from build123d import *

# Parameters (mm, degrees)
SKETCH1_R           = 15
SKETCH1_R_2         = 10.05
BOSS_EXTRUDE1_DEPTH = 6
SKETCH3_R           = 2.95
CUT_EXTRUDE1_DEPTH  = 3
CIRPATTERN1_COUNT   = 3
SKETCH4_R           = 1.65
CUT_EXTRUDE2_DEPTH  = 11
CIRPATTERN3_COUNT   = 3


with BuildPart() as part:
    # Sketch1 → Boss-Extrude1 (new body)
    with BuildSketch(Plane(origin=(0, 0, 0), x_dir=(0, 0, -1), z_dir=(1, 0, 0))):
        Circle(SKETCH1_R)
        Circle(SKETCH1_R_2, mode=Mode.SUBTRACT)
    extrude(amount=BOSS_EXTRUDE1_DEPTH)

    # Sketch3 → Cut-Extrude1 (cut)
    with BuildSketch(Plane(origin=(0, -7.5, 12.990381057), x_dir=(1, 0, 0), z_dir=(0, -0.5000000000000044, 0.866025403784436))):
        with Locations(Location((3, 0, 0), (0, 0, 270))):
            Circle(SKETCH3_R)
    cut_extrude1 = extrude(amount=-CUT_EXTRUDE1_DEPTH, mode=Mode.SUBTRACT)

    # CirPattern1: Cut-Extrude1 ×3 about axis
    cirpattern1_axis = Axis((0, 0, 0), (1, 0, 0))
    for i in range(1, CIRPATTERN1_COUNT):
        add(cut_extrude1.rotate(cirpattern1_axis, i * 360 / CIRPATTERN1_COUNT), mode=Mode.SUBTRACT)

    # Sketch4 → Cut-Extrude2 (cut)
    with BuildSketch(Plane(origin=(0, -7.5, 12.990381057), x_dir=(1, 0, 0), z_dir=(0, -0.5000000000000044, 0.866025403784436))):
        with Locations(Location((3, 0, 0), (0, 0, 270))):
            Circle(SKETCH4_R)
    cut_extrude2 = extrude(amount=-CUT_EXTRUDE2_DEPTH, mode=Mode.SUBTRACT)

    # CirPattern3: Cut-Extrude2 ×3 about axis
    cirpattern3_axis = Axis((6, 0, 0), (-1, 0, 0))
    for i in range(1, CIRPATTERN3_COUNT):
        add(cut_extrude2.rotate(cirpattern3_axis, i * 360 / CIRPATTERN3_COUNT), mode=Mode.SUBTRACT)


solid = part.part
Verification items for the finished model (mm, model axes). A direction names the side the tool comes from. Coordinates: 2 decimals unless noted, no trailing zeros. Order: outer loops, then holes, each group sorted by start corner. A loop starts at its lowest first (then second) coordinate and runs counter-clockwise, first axis right, second up. Notation, with made-up numbers: (27.5, 78) -> (69.5, 78) arc R35 ccw to (69.5, 111) -> close; hole circle Ø10 at (60, -30.5). An arc over 180 degrees is marked (long way). Put each result on its own line as item: value. Start each with the question number.
1. Go/stop test with flat-tipped pins: pin 1 Ø3.5 at (x, z) = (3, 0) entering from +Y; pin 2 Ø2 at (x, z) = (3, -9) entering from -Y; pin 3 Ø2 at (x, z) = (5.5, 10) entering from -Y. Record where each tip stops, or that it passes through.
2. Mould release check, pull along X, two halves, no side actions. Record for faces 1 (the cylindrical face through (3.496, -6.848, 8.713)), 2 (the flat face through (6, -10, -3)), 3 (the flat face through (0, -10, -3)): released by +X, released by -X, zero draft, split by the parting line, or undercut.
3. Access from +Z, -Z, +X, -X, +Y, -Y to the whole of each face (thin tool, end or side, straight path). Record for faces 4 (the flat face through (1.07, -6.04, -10.37)), 5 (the cylindrical face through (2.96, -9.81, 2.18)), 6 (the cylindrical face through (3.886, 13.521, 2.814)).
4. Material ranges on L1, parallel to Y at x = 3.5, z = 0; L2, parallel to Y at x = 3.5, z = 11; L3, parallel to X at y = -8.5, z = 10.5, recorded low to high. Write a range as [from, to].
5. Cross-section at B-B, the plane z = 0. Record the boundary of the cut face in (x, y).
6. Cross-section at A-A, the plane y = 0. Record the boundary of the cut face in (x, z).
7. Cross-section at D-D, the plane z = -5.5. Record the boundary of the cut face in (x, y), then the cut area to 3 significant figures.
8. Cross-section at C-C, the plane x = 3. Record the boundary of the cut face in (y, z).
Computed:
1. pin 1: y = 12
1. pin 2: y = -12.69
1. pin 3: y = -12
2. face 1: undercut
2. face 2: released by +X
2. face 3: released by -X
3. face 4: none
3. face 5: +X, -X
3. face 6: +Y
4. L1: [-15, -10.05]
4. L2: [-10.2, -9.71], [-4.54, 10.2]
4. L3: [0, 0.94], [5.06, 6]
5. outline: (0, -15) -> (6, -15) -> (6, -10.05) -> (0, -10.05) -> close; (0, 10.05) -> (1.35, 10.05) -> (1.35, 12) -> (0.05, 12) -> (0.05, 15) -> (0, 15) -> close; (4.65, 10.05) -> (6, 10.05) -> (6, 15) -> (5.95, 15) -> (5.95, 12) -> (4.65, 12) -> close
6. outline: (0, -15) -> (6, -15) -> (6, -10.05) -> (0, -10.05) -> close; (0, 10.05) -> (6, 10.05) -> (6, 15) -> (0, 15) -> close
7. outline: (0, -13.96) -> (6, -13.96) -> (6, -8.41) -> (0, -8.41) -> close; (0, 8.41) -> (6, 8.41) -> (6, 13.96) -> (0, 13.96) -> close
7. area: 66.5 mm2
8. outline: (-9.91, -11.26) -> (-8.55, -8.92) -> (-7.43, -9.57) -> (-6.39, -7.76) arc R10.05 cw to (-6.39, 7.76) -> (-7.43, 9.57) -> (-8.55, 8.92) -> (-9.91, 11.26) arc R15 ccw to start; (-4.8, -14.21) arc R15 ccw to (14.71, -2.95) -> (12, -2.95) -> (12, -1.65) -> (9.91, -1.65) arc R10.05 cw to (-3.53, -9.41) -> (-4.57, -11.22) -> (-3.45, -11.87) -> close; (-4.8, 14.21) -> (-3.45, 11.87) -> (-4.57, 11.22) -> (-3.53, 9.41) arc R10.05 cw to (9.91, 1.65) -> (12, 1.65) -> (12, 2.95) -> (14.71, 2.95) arc R15 ccw to start
